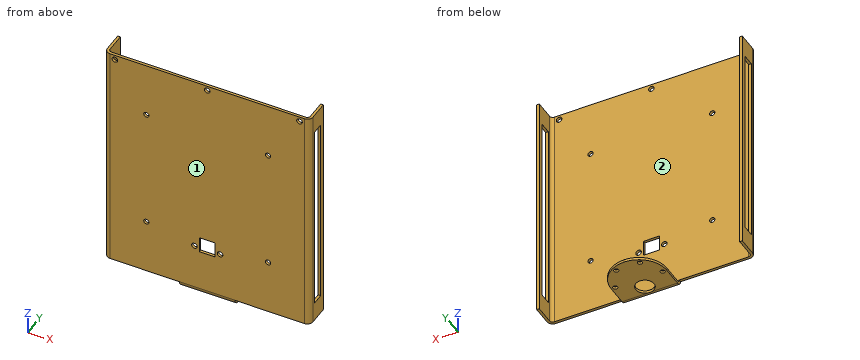
from build123d import *

# Parameters (mm, degrees)
F1_DEPTH  = 152.4
F2_W      = 7.9375
F2_H      = 127.0931567346
F3_DEPTH  = 134.38632
F4_W      = 36.322
F4_H      = 1.70942
F5_DEPTH  = 3.69316
F6_W      = 36.322
F6_H      = 1.70942
F7_DEPTH  = 33.4645
F8_R      = 3.69316
F9_R      = 1.98374
F10_R     = 5.969
F10_R_2   = 1.5
F11_DEPTH = 3.69316
F12_R     = 18.16099
F13_R     = 1.8288
F14_DEPTH = 1.70942
F15_R     = 1.7272
F16_DEPTH = 1.70942
F17_W     = 10.40892
F17_H     = 10.40892
F17_R     = 1.8288
F18_DEPTH = 1.70942


# Not quite as in the source:
# - a fillet or chamfer is up to 0.001 mm smaller than in the source, because OpenCascade refuses the exact size


with BuildPart() as f1:
    # F0 (on Top) → F1 (new body)
    with BuildSketch(Plane.XY):
        Polygon((0, 14.68374), (0, 0), (-130.96748, 0), (-130.96748, 14.68374), (-132.6769, 14.68374), (-132.6769, -1.70942), (1.70942, -1.70942), (1.70942, 14.68374), align=None)
    extrude(amount=F1_DEPTH)

    # F2 (on face) → F3 (cut, through all)
    with BuildSketch(Plane.YZ.offset(1.70942)):
        with Locations((7.53999, 76.2)):
            Rectangle(F2_W, F2_H)
    extrude(amount=-F3_DEPTH, mode=Mode.SUBTRACT)

    # F4 (on face) → F5 (join)
    with BuildSketch(Plane(origin=(0, 0, 0), x_dir=(1, 0, 0), z_dir=(0, 0, -1))):
        with Locations((-65.48374, 0.85471)):
            Rectangle(F4_W, F4_H)
    extrude(amount=F5_DEPTH)

    # F6 (on face) → F7 (join)
    with BuildSketch(Plane(origin=(0, 0, 0), x_dir=(-1, 0, 0), z_dir=(0, 1, 0))):
        with Locations((65.48374, -2.83845)):
            Rectangle(F6_W, F6_H)
    extrude(amount=F7_DEPTH)

    # F8
    f8_edges = [f1.edges().sort_by_distance(p)[0] for p in [
        (1.70942, -1.70942, 76.2),
        (-132.6769, -1.70942, 76.2),
        (-65.48374, -1.70942, -3.69316),
    ]]
    fillet(f8_edges, radius=F8_R)

    # F9
    f9_edges = [f1.edges().sort_by_distance(p)[0] for p in [
        (0, 0, 76.2),
        (-130.96748, 0, 76.2),
        (-65.48374, 0, -1.98374),
    ]]
    fillet(f9_edges, radius=F9_R)

    # F10 (on face) → F11 (cut, through all)
    with BuildSketch(Plane(origin=(0, 0, -3.69316), x_dir=(1, 0, 0), z_dir=(0, 0, -1))):
        with Locations((-65.48374, -7.9375)):
            Circle(F10_R)
        with Locations((-49.9897398917, -15.3035)):
            Circle(F10_R_2)
        with Locations((-80.9777401083, -15.3035)):
            Circle(F10_R_2)
        with Locations((-73.2307400541, -28.7216977)):
            Circle(F10_R_2)
        with Locations((-57.7367399459, -28.7216977)):
            Circle(F10_R_2)
    extrude(amount=-F11_DEPTH, mode=Mode.SUBTRACT)

    # F12 (radius 18.161 in the source; OpenCascade refuses exactly that, so slightly less here)
    f12_edges = [f1.edges().sort_by_distance(p)[0] for p in [
        (-47.32274, 33.4645, -2.83845),
        (-83.64474, 33.4645, -2.83845),
    ]]
    fillet(f12_edges, radius=F12_R)

    # F13 (on face) → F14 (cut, through all)
    with BuildSketch(Plane.XZ.offset(1.70942)):
        with Locations((-65.48374, 149.225)):
            Circle(F13_R)
        with Locations((-5.15874, 149.225)):
            Circle(F13_R)
        with Locations((-125.80874, 149.225)):
            Circle(F13_R)
    extrude(amount=-F14_DEPTH, mode=Mode.SUBTRACT)

    # F15 (on face) → F16 (cut, through all)
    with BuildSketch(Plane.XZ.offset(1.70942)):
        with Locations((-105.2585017, 115.9747617)):
            Circle(F15_R)
        with Locations((-25.7089783, 115.9747617)):
            Circle(F15_R)
        with Locations((-25.7089783, 36.4252383)):
            Circle(F15_R)
        with Locations((-105.2585017, 36.4252383)):
            Circle(F15_R)
    extrude(amount=-F16_DEPTH, mode=Mode.SUBTRACT)

    # F17 (on face) → F18 (cut, through all)
    with BuildSketch(Plane(origin=(0, 0, 0), x_dir=(-1, 0, 0), z_dir=(0, 1, 0))):
        with Locations((65.48374, 32.4986058015)):
            Rectangle(F17_W, F17_H)
        with Locations((73.8632, 30.4691458015)):
            Circle(F17_R)
        with Locations((57.10428, 30.4691458015)):
            Circle(F17_R)
    extrude(amount=-F18_DEPTH, mode=Mode.SUBTRACT)


solid = f1.part
Work out the finished part from the listing and answer in its coordinate system (mm). Face numbers are marked on the shaded views. A direction names the side the tool comes from. Coordinates: 2 decimals unless noted, no trailing zeros. Loops run counter-clockwise (first coordinate to the right, second up) from the corner with the lowest first, then second, coordinate; pieces in that order, holes last. Notation, with made-up numbers: (12.25, -6.5) -> (36.25, -6.5) arc R11 ccw to (36.25, -1.5) -> close; hole circle Ø5 at (19.25, -2). An arc over 180 degrees is marked (long way). Write each question's results on one line, items separated by ' | '. Start each with the question number.
1) Find section B-B on x = -31. Determine the outline of the cut face in (y, z), then the cut area to 3 significant figures.
2) For the marked faces 1 and 2, determine the directions among +Z, -Z, +X, -X, +Y, -Y from which every point of the face is accessible in a straight line to the end or side of a thin tool.
3) Find section A-A on z = 95. Determine the outline of the cut face in (x, y), then the cut area to 3 significant figures.
4) Flat-ended cylindrical pins translate along their axes: P1, Ø12, axis at y = 15, z = 113, coming from the +X side; P2, Ø1.4, axis at x = -132, z = 60, coming from the -Y side; P3, Ø6, axis at x = -49.5, z = 128, coming from the +Y side; P4, Ø1.4, axis at x = -132, z = 69.5, coming from the +Y side. Find the tip coordinate at first contact, or state that the pin passes through.
5) Find section C-C on y = 21. Determine the outline of the cut face in (x, z), then the cut area to 3 significant figures.
6) Consider line 1 along X through (y, z) = (14, 136.5); line 2 along Y through (x, z) = (-69.5, 102.5); line 3 along X through (y, z) = (0.5, 127). Determine where each line is inside the solid, lowest interval first.
Response values:
1) outline: (-1.71, 0) -> (0, 0) -> (0, 152.4) -> (-1.71, 152.4) -> close | area: 261 mm^2
2) face 1: +Z, -Z, +X, -X, -Y | face 2: +Z, +Y
3) outline: (-132.68, 1.98) arc R3.69 ccw to (-128.98, -1.71) -> (-1.98, -1.71) arc R3.69 ccw to (1.71, 1.98) -> (1.71, 3.57) -> (0, 3.57) -> (0, 1.98) arc R1.98 cw to (-1.98, 0) -> (-128.98, 0) arc R1.98 cw to (-130.97, 1.98) -> (-130.97, 3.57) -> (-132.68, 3.57) -> close; (-132.68, 11.51) -> (-130.97, 11.51) -> (-130.97, 14.68) -> (-132.68, 14.68) -> close; (0, 11.51) -> (1.71, 11.51) -> (1.71, 14.68) -> (0, 14.68) -> close | area: 249 mm^2
4) P1: stops at x = 1.71 | P2: stops at y = -0.89 | P3: stops at y = 0 | P4: stops at y = 14.68
5) outline: (-82.73, -3.69) -> (-48.24, -3.69) -> (-48.24, -1.98) -> (-82.73, -1.98) -> close | area: 59.0 mm^2
6) line 1: x = -132.68 to -130.97, 0 to 1.71 | line 2: y = -1.71 to 0 | line 3: x = -132.37 to -130.3, -0.67 to 1.4
